Answer from the drawing. Dimensions are ordinates in mm from the lowest x, y and z of the part. A direction names the side the tool comes from. Coordinates: 2 decimals unless noted, no trailing zeros. Write each loop counter-clockwise with the first axis right and the second up, starting at its lowest first coordinate (ties: lowest second). Pieces come first, ordered by that corner, then holes.
(1) Given pin 1 (1 mm diameter, centred on x = 1, z = 1.5, fed in from -Y), flat-ended and moving along its own axis, determine where the tip first touches the part or whether it passes through.
(2) Which of the six approach directions +Z, -Z, +X, -X, +Y, -Y give full straight-line access (tool end or side, diameter ignored) to the marked faces 3 and 4?
(3) The part is cut by section A-A, the plane y = 2.75. Determine the outline of the cut face in (x, z).
(4) The part is cut by section C-C, the plane z = 9. Determine the outline of the cut face in (x, y).
(5) Straight lines are drawn through the part: line 1 along Y through (x, z) = (1.8, 3.25); line 2 along Z through (x, y) = (3.55, 4.7); line 3 along X through (y, z) = (2.2, 2.25). For each, find the intervals that lie inside material, in ascending order.
(6) Determine the mould class of the marked faces 1 and 2 for opening direction X: pulls with the +X half, pulls with the -X half, needs draft (parallel to the pull), parting line crosses it, or undercut.
(7) The part is cut by section D-D, the plane z = 10.75. Determine the outline of the cut face in (x, y), and give its area (3 significant figures).
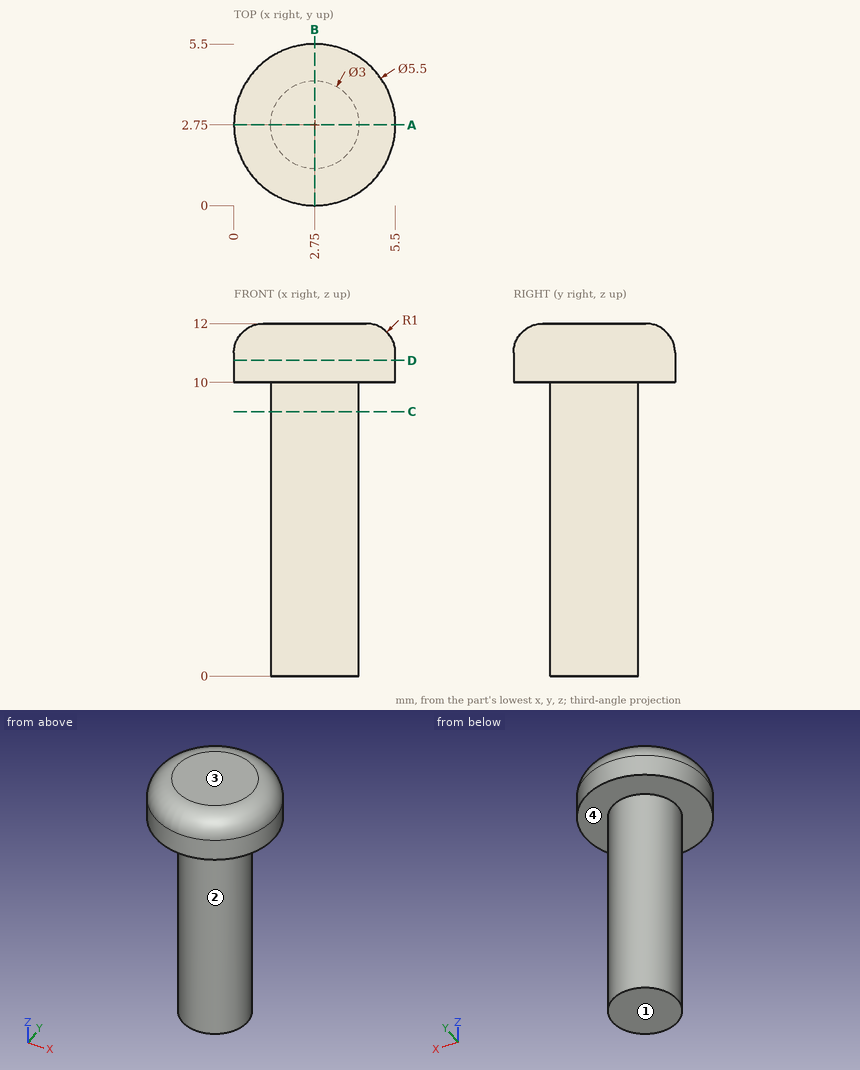
Computed:
1. pin 1: stops at y = 1.92
2. face 3: +Z, +X, -X, +Y, -Y
2. face 4: -Z
3. outline: (0, 10) - (1.25, 10) - (1.25, 0) - (4.25, 0) - (4.25, 10) - (5.5, 10) - (5.5, 11) arc R1 ccw to (4.5, 12) - (1, 12) arc R1 ccw to (0, 11) - close
4. outline: circle Ø3 at (2.75, 2.75)
5. line 1: y = 1.59 to 3.91
5. line 2: z = 10 to 11.93
5. line 3: x = 1.35 to 4.15
6. face 1: needs draft
6. face 2: parting line crosses it
7. outline: circle Ø5.5 at (2.75, 2.75)
7. area: 23.8 mm2
